Geometry: final body of the model. Coordinates: model frame, mm. A direction names the side the tool comes from. Give positions to 0.01 mm unless a question says otherwise; leave off trailing zeros. Loops run counter-clockwise (first coordinate to the right, second up) from the corner with the lowest first, then second, coordinate; pieces in that order, holes last.
1. Draft query along Z for faces 5 (the face through (-28.329, 25, -45)), 6 (the face through (6, 26, 24.073)), 7 (the face through (-45, 22, 19.073)). Return one class per face: +Z half, -Z half, draft (parallel to the pull), parting line (faces both ways), or undercut.
2. Material intervals for line 1 along Z through (x, y) = (-42, 13); line 2 along X through (y, z) = (46, 4); line 3 along Y through (x, z) = (8, -23), sorted ascending.
3. Section C-C, the plane y = 46. Output: boundary loops of the cut face in (x, z).
4. Access query for faces 1 (the face through (66, 26, 21.073)), 2 (the face through (45, 18, -40)), 3 (the face through (-47, 13, 14)), 4 (the face through (4, 28, -38.927)). Directions: +Z, -Z, +X, -X, +Y, -Y. A direction counts if a zero-diameter tool reaches every point of the face in a straight line with its end or side. Return the directions, or none.
5. First-contact query: P1, Ø5, axis at y = 35, z = -13, coming from the -X side; P2, Ø2, axis at y = 28, z = -38.5, coming from the +X side; P3, Ø12, axis at x = -16, z = 12.5, coming from the +Y side. Flat tips, straight axial feed; report the tip coordinate or a pass-through.
6. Section A-A, the plane z = 17.5. Output: boundary loops of the cut face in (x, y), then the cut area to 3 significant figures.
7. Section D-D, the plane y = 10. State how many separate pieces and enclosed holes the cut face has, then the cut area to 3 significant figures.
8. Section B-B, the plane x = -41. Output: boundary loops of the cut face in (y, z), then the cut area to 3 significant figures.
from build123d import *

# Parameters (mm, degrees)
CROQUIS1_W                   = 100
CROQUIS1_H                   = 60
SALIENTE_EXTRUIR1_DEPTH      = 3
SALIENTE_EXTRUIR2_DEPTH      = 50
SALIENTE_EXTRUIR2_DEPTH_BACK = 3
CROQUIS2_W                   = 106
CROQUIS2_H                   = 66
CROQUIS2_W_2                 = 100
CROQUIS2_H_2                 = 60
CROQUIS3_W                   = 2
CROQUIS3_H                   = 2
SALIENTE_EXTRUIR3_DEPTH      = 50
CROQUIS4_W                   = 30
CROQUIS4_H                   = 20
CROQUIS4_W_2                 = 10
CROQUIS4_H_2                 = 10
CORTAR_EXTRUIR2_DEPTH        = 24
CROQUIS5_W                   = 30
CROQUIS5_H                   = 30
CROQUIS5_W_2                 = 26
CROQUIS5_H_2                 = 26
SALIENTE_EXTRUIR4_DEPTH      = 6
CROQUIS6_W                   = 2
CROQUIS6_H                   = 2
CORTAR_EXTRUIR3_DEPTH        = 6
CROQUIS7_W                   = 15
CROQUIS7_H                   = 15
CORTAR_EXTRUIR4_DEPTH        = 6
CROQUIS8_R                   = 1
CORTAR_EXTRUIR5_DEPTH        = 53
CROQUIS9_W                   = 3
CROQUIS9_H                   = 53
SALIENTE_EXTRUIR5_DEPTH      = 10
CROQUIS10_W                  = 3
CROQUIS10_H                  = 53
SALIENTE_EXTRUIR6_DEPTH      = 10
CROQUIS12_R                  = 2.5
CORTAR_EXTRUIR6_DEPTH        = 10


with BuildPart() as part:
    # Croquis1 → Saliente-Extruir1 (new body)
    with BuildSketch(Plane(origin=(0, 0, 0), x_dir=(1, 0, 0), z_dir=(0, 1, 0))):
        with Locations((4.671280277, 8.92733564)):
            Rectangle(CROQUIS1_W, CROQUIS1_H)
    extrude(amount=SALIENTE_EXTRUIR1_DEPTH)

    # Croquis2 → Saliente-Extruir2 (add, two sides: drawn at the far end of the back side and taken through both)
    with BuildSketch(Plane(origin=(0, 3, 0), x_dir=(1, 0, 0), z_dir=(0, 1, 0)).offset(-SALIENTE_EXTRUIR2_DEPTH_BACK)):
        with Locations((4.671280277, 8.92733564)):
            Rectangle(CROQUIS2_W, CROQUIS2_H)
        with Locations((4.671280277, 8.92733564)):
            Rectangle(CROQUIS2_W_2, CROQUIS2_H_2, mode=Mode.SUBTRACT)
    extrude(amount=SALIENTE_EXTRUIR2_DEPTH + SALIENTE_EXTRUIR2_DEPTH_BACK)

    # Croquis3 → Saliente-Extruir3 (add)
    with BuildSketch(Plane(origin=(0, 3, 0), x_dir=(1, 0, 0), z_dir=(0, 1, 0))):
        with Locations((-44.328719723, 37.92733564)):
            Rectangle(CROQUIS3_W, CROQUIS3_H)
        with Locations((-44.328719723, -20.07266436)):
            Rectangle(CROQUIS3_W, CROQUIS3_H)
        with Locations((53.671280277, -20.07266436)):
            Rectangle(CROQUIS3_W, CROQUIS3_H)
        with Locations((53.671280277, 37.92733564)):
            Rectangle(CROQUIS3_W, CROQUIS3_H)
    extrude(amount=SALIENTE_EXTRUIR3_DEPTH)

    # Croquis4 → Cortar-Extruir2 (cut)
    with BuildSketch(Plane.ZY.offset(48.328719723)):
        with Locations((-21.92733564, 13)):
            Rectangle(CROQUIS4_W, CROQUIS4_H)
        with Locations((14.07266436, 8)):
            Rectangle(CROQUIS4_W_2, CROQUIS4_H_2)
    extrude(amount=-CORTAR_EXTRUIR2_DEPTH, mode=Mode.SUBTRACT)

    # Croquis5 → Saliente-Extruir4 (add)
    with BuildSketch(Plane(origin=(0, 0, -41.92733564), x_dir=(-1, 0, 0), z_dir=(0, 0, -1))):
        with Locations((15.328719723, 18)):
            Rectangle(CROQUIS5_W, CROQUIS5_H)
        with Locations((15.328719723, 18)):
            Rectangle(CROQUIS5_W_2, CROQUIS5_H_2, mode=Mode.SUBTRACT)
    extrude(amount=SALIENTE_EXTRUIR4_DEPTH)

    # Croquis6 → Cortar-Extruir3 (cut)
    with BuildSketch(Plane(origin=(0, 0, -47.92733564), x_dir=(-1, 0, 0), z_dir=(0, 0, -1))):
        with Locations((29.328719723, 18)):
            Rectangle(CROQUIS6_W, CROQUIS6_H)
    extrude(amount=-CORTAR_EXTRUIR3_DEPTH, mode=Mode.SUBTRACT)

    # Croquis7 → Cortar-Extruir4 (cut)
    with BuildSketch(Plane(origin=(0, 0, -41.92733564), x_dir=(-1, 0, 0), z_dir=(0, 0, -1))):
        with Locations((-45.171280277, 10.5)):
            Rectangle(CROQUIS7_W, CROQUIS7_H)
    extrude(amount=-CORTAR_EXTRUIR4_DEPTH, mode=Mode.SUBTRACT)

    # Croquis8 → Cortar-Extruir5 (cut)
    with BuildSketch(Plane(origin=(0, 53, 0), x_dir=(1, 0, 0), z_dir=(0, 1, 0))):
        with Locations(Location((-45.828719723, 39.42733564, 0), (0, 0, 270))):
            Circle(CROQUIS8_R)
        with Locations(Location((55.171280277, 39.42733564, 0), (0, 0, 270))):
            Circle(CROQUIS8_R)
        with Locations(Location((55.171280277, -21.57266436, 0), (0, 0, 270))):
            Circle(CROQUIS8_R)
        with Locations(Location((-45.828719723, -21.57266436, 0), (0, 0, 270))):
            Circle(CROQUIS8_R)
    extrude(amount=-CORTAR_EXTRUIR5_DEPTH, mode=Mode.SUBTRACT)

    # Croquis9 → Saliente-Extruir5 (add)
    with BuildSketch(Plane(origin=(57.671280277, 0, 0), x_dir=(0, 0, -1), z_dir=(1, 0, 0))):
        with Locations((-22.57266436, 26.5)):
            Rectangle(CROQUIS9_W, CROQUIS9_H)
    extrude(amount=SALIENTE_EXTRUIR5_DEPTH)

    # Croquis10 → Saliente-Extruir6 (add)
    with BuildSketch(Plane.ZY.offset(48.328719723)):
        with Locations((22.57266436, 26.5)):
            Rectangle(CROQUIS10_W, CROQUIS10_H)
    extrude(amount=SALIENTE_EXTRUIR6_DEPTH)

    # Croquis12 → Cortar-Extruir6 (cut)
    with BuildSketch(Plane(origin=(0, 0, 21.07266436), x_dir=(-1, 0, 0), z_dir=(0, 0, -1))):
        with Locations(Location((-62.671280277, 26.5, 0), (0, 0, 90))):
            Circle(CROQUIS12_R)
        with Locations(Location((53.328719723, 26.5, 0), (0, 0, 90))):
            Circle(CROQUIS12_R)
    extrude(amount=-CORTAR_EXTRUIR6_DEPTH, mode=Mode.SUBTRACT)


solid = part.part
Answers below:
1. face 5: draft
1. face 6: +Z half
1. face 7: undercut
2. line 1: z = -41.93 to -38.93, 21.07 to 24.07
2. line 2: x = -48.33 to -45.33, 54.67 to 57.67
2. line 3: y = 0 to 3
3. outline: (-58.33, 21.07) - (-48.33, 21.07) - (-48.33, -41.93) - (57.67, -41.93) - (57.67, 21.07) - (67.67, 21.07) - (67.67, 24.07) - (-58.33, 24.07) - close; hole circle Ø2 at (-45.83, -39.43); hole circle Ø2 at (-45.83, 21.57); hole (-45.33, -36.93) - (-43.33, -36.93) - (-43.33, -38.93) - (52.67, -38.93) - (52.67, -36.93) - (54.67, -36.93) - (54.67, 19.07) - (52.67, 19.07) - (52.67, 21.07) - (-43.33, 21.07) - (-43.33, 19.07) - (-45.33, 19.07) - close; hole circle Ø2 at (55.17, -39.43); hole circle Ø2 at (55.17, 21.57)
4. face 1: -Z, +X, +Y, -Y
4. face 2: -Z
4. face 3: -X
4. face 4: +Y
5. P1: stops at x = -48.33
5. P2: stops at x = 57.67
5. P3: stops at y = 3
6. outline: (-48.33, 0) - (57.67, 0) - (57.67, 53) - (54.67, 53) - (54.67, 3) - (-48.33, 3) - close; (-48.33, 13) - (-45.33, 13) - (-45.33, 53) - (-48.33, 53) - close
6. area: 588 mm2
7. separate pieces: 3
7. enclosed holes: 4
7. area: 918 mm2
8. outline: (0, -41.93) - (53, -41.93) - (53, -38.93) - (3, -38.93) - (3, 21.07) - (53, 21.07) - (53, 24.07) - (0, 24.07) - close
8. area: 498 mm2
